Model file for the job. Use its own axes, mm. Face numbers are marked on the shaded views. Coordinates: 2 decimals unless noted, no trailing zeros. Order: outer loops, then holes, each group sorted by start corner. A loop starts at its lowest first (then second) coordinate and runs counter-clockwise, first axis right, second up. Notation, with made-up numbers: (72.25, 32) -> (86.25, 32) arc R17 ccw to (86.25, 52) -> close; hole circle Ø6 at (89, 35). An arc over 180 degrees is marked (long way). Write item = value, one per line. Start each with the question number.
Q1. Flat gauge pins, fed straight in: pin 1 (1 mm diameter, centred on x = 2, y = 3, fed in from -Z); pin 2 (1.5 mm diameter, centred on x = 0, z = 0, fed in from -Y). Where does each tip first touch, or does it go through?
Q2. Cut at C-C, the plane y = 1.95. List the corners of the cut face in (x, z), plus the area to 3 significant figures.
Q3. Cut at B-B, the plane z = 1.5. List the corners of the cut face in (x, y).
Q4. Wall check: line 1 (Y direction, x = 2, z = 1.1); line 2 (X direction, y = 4.8, z = -0.5); line 3 (Z direction, x = 0.3, y = 2.6). Give the ranges that are in metal, low to high. Write a range as from..to.
Q5. Mould opens along Z. For the marked faces 1, 2 and 3 say: +Z half, -Z half, draft (parallel to the pull), parting line (faces both ways), or undercut.
Q6. Cut at D-D, the plane z = -0.65. List the corners of the cut face in (x, y).
Q7. Cut at A-A, the plane z = 0.1. List the corners of the cut face in (x, y), plus the area to 3 significant figures.
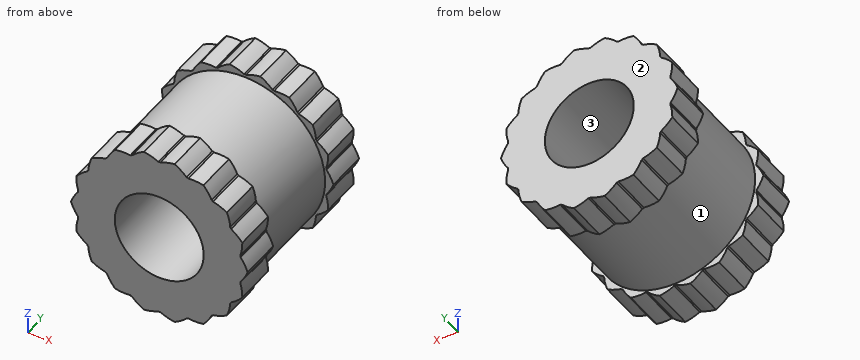
from build123d import *

# Parameters (mm, degrees)
SKETCH1_R           = 2.51
BOSS_EXTRUDE1_DEPTH = 5
CUT_EXTRUDE2_DEPTH  = 5
CIRPATTERN1_COUNT   = 18
M3_TAPPED_HOLE1_D   = 2.5
SKETCH8_R           = 3.25
SKETCH8_R_2         = 2.25
CUT_EXTRUDE3_DEPTH  = 2.7


with BuildPart() as part:
    # Sketch1 → Boss-Extrude1 (new body)
    with BuildSketch(Plane(origin=(0, 0, 0), x_dir=(1, 0, 0), z_dir=(0, 1, 0))):
        with Locations(Location((0, 0, 0), (0, 0, 270))):
            Circle(SKETCH1_R)
    extrude(amount=BOSS_EXTRUDE1_DEPTH)

    # Sketch2 → Cut-Extrude2 (cut)
    with BuildSketch(Plane(origin=(0, 5, 0), x_dir=(1, 0, 0), z_dir=(0, 1, 0))):
        with BuildLine():
            ThreePointArc((0.569091169, 2.444633969), (0, 2.615621061), (-0.569091169, 2.444633969))
            ThreePointArc((-0.569091169, 2.444633969), (-0.289139314, 2.403802024), (-0.024469936, 2.303849986))
            ThreePointArc((-0.024469936, 2.303849986), (0, 2.310246979), (0.024469936, 2.303849986))
            ThreePointArc((0.024469936, 2.303849986), (0.289139314, 2.403802024), (0.569091169, 2.444633969))
        make_face()
    cut_extrude2 = extrude(amount=-CUT_EXTRUDE2_DEPTH, mode=Mode.SUBTRACT)

    # CirPattern1: Cut-Extrude2 ×18 about axis
    cirpattern1_axis = Axis((0, 0, 0.013606971), (0, 1, 0))
    for i in range(1, CIRPATTERN1_COUNT):
        add(cut_extrude2.rotate(cirpattern1_axis, i * 360 / CIRPATTERN1_COUNT), mode=Mode.SUBTRACT)

    # M3 Tapped Hole1 (through all)
    with Locations(Plane(origin=(0, 5, 0), x_dir=(1, 0, 0), z_dir=(0, 1, 0))):
        with Locations((0, 0)):
            Hole(M3_TAPPED_HOLE1_D / 2)

    # Sketch8 → Cut-Extrude3 (cut)
    with BuildSketch(Plane(origin=(0, 3.85, 0), x_dir=(1, 0, 0), z_dir=(0, 1, 0))):
        Circle(SKETCH8_R)
        with Locations(Location((0, 0, 0), (0, 0, 270))):
            Circle(SKETCH8_R_2, mode=Mode.SUBTRACT)
    extrude(amount=-CUT_EXTRUDE3_DEPTH, mode=Mode.SUBTRACT)


solid = part.part
Here are the results:
q1.pin_1 = -1.68
q1.pin_2 = through
q2.outline = circle Ø4.5 at (0, 0); hole circle Ø2.5 at (0, 0)
q2.area = 11.0 mm²
q3.outline = (-1.94, 0) -> (1.94, 0) -> (1.94, 1.15) -> (1.68, 1.15) -> (1.68, 3.85) -> (1.94, 3.85) -> (1.94, 5) -> (-1.94, 5) -> (-1.94, 3.85) -> (-1.68, 3.85) -> (-1.68, 1.15) -> (-1.94, 1.15) -> close
q4.line_1 = 0..1.15, 3.85..5
q4.line_2 = -2.3..-1.15, 1.15..2.3
q4.line_3 = -2.23..-1.21, 1.21..2.23
q5.face_1 = parting line
q5.face_2 = draft
q5.face_3 = undercut
q6.outline = (-2.33, 0) -> (-1.07, 0) -> (-1.07, 5) -> (-2.33, 5) -> (-2.33, 3.85) -> (-2.15, 3.85) -> (-2.15, 1.15) -> (-2.33, 1.15) -> close; (1.07, 0) -> (2.33, 0) -> (2.33, 1.15) -> (2.15, 1.15) -> (2.15, 3.85) -> (2.33, 3.85) -> (2.33, 5) -> (1.07, 5) -> close
q7.outline = (-2.45, 0) -> (-1.25, 0) -> (-1.25, 5) -> (-2.45, 5) -> (-2.45, 3.85) -> (-2.25, 3.85) -> (-2.25, 1.15) -> (-2.45, 1.15) -> close; (1.25, 0) -> (2.45, 0) -> (2.45, 1.15) -> (2.25, 1.15) -> (2.25, 3.85) -> (2.45, 3.85) -> (2.45, 5) -> (1.25, 5) -> close
q7.area = 11.0 mm²
